from build123d import *

# Parameters (mm, degrees)
BOSS_EXTRUDE1_DEPTH      = 5
BOSS_EXTRUDE1_DEPTH_BACK = 5
SKETCH1_R                = 1.5
CUT_EXTRUDE1_DEPTH       = 5
SKETCH5_R                = 2.5
CUT_EXTRUDE3_DEPTH       = 30
SKETCH6_R                = 1.5
SKETCH6_R_2              = 1.843261337
CUT_EXTRUDE4_DEPTH       = 42


with BuildPart() as part:
    # Sketch1 → Boss-Extrude1 (new, two sides: drawn at the far end of the back side and taken through both)
    with BuildSketch(Plane(origin=(0, 0, 0), x_dir=(1, 0, 0), z_dir=(0, 1, 0)).offset(-BOSS_EXTRUDE1_DEPTH_BACK)):
        with BuildLine():
            Line((0, 17.525), (0, 40))
            Line((0, 40), (-36, 40))
            Line((-36, 40), (-36, -40))
            Line((-36, -40), (0, -40))
            Line((0, -40), (0, -17.525))
            ThreePointArc((0, -17.525), (-17.525, 0), (0, 17.525))
        make_face()
        with Locations(Location((-24.748737342, 24.748737342, 0), (0, 0, 270))):
            Circle(SKETCH1_R, mode=Mode.SUBTRACT)
        with Locations(Location((-24.748737342, -24.748737342, 0), (0, 0, 270))):
            Circle(SKETCH1_R, mode=Mode.SUBTRACT)
    extrude(amount=BOSS_EXTRUDE1_DEPTH + BOSS_EXTRUDE1_DEPTH_BACK)

    # Sketch2 → Cut-Extrude1 (cut)
    with BuildSketch(Plane(origin=(0, 5, 0), x_dir=(1, 0, 0), z_dir=(0, 1, 0))):
        Polygon((-23.161024101, 27.498737342), (-26.336450582, 27.498737342), (-27.924163822, 24.748737342), (-26.336450582, 21.998737342), (-23.161024101, 21.998737342), (-21.573310861, 24.748737342), align=None)
    cut_extrude1 = extrude(amount=-CUT_EXTRUDE1_DEPTH, mode=Mode.SUBTRACT)

    # Mirror1: Cut-Extrude1 across plane
    add(cut_extrude1.mirror(Plane.XY), mode=Mode.SUBTRACT)

    # Sketch5 → Cut-Extrude3 (cut)
    with BuildSketch(Plane.ZY.offset(36)):
        with Locations((-30, 0)):
            Circle(SKETCH5_R)
        Polygon((31.592573026, 2.747490689), (28.417151509, 2.753105152), (26.824578483, 0.005916682), (28.407426974, -2.746886251), (31.582848491, -2.752500714), (33.175421517, -0.005312244), align=None)
    extrude(amount=-CUT_EXTRUDE3_DEPTH, mode=Mode.SUBTRACT)

    # Sketch6 → Cut-Extrude4 (cut)
    with BuildSketch(Plane.ZY.offset(36)):
        with Locations((-30, 0)):
            Circle(SKETCH6_R)
        with Locations((30, 0)):
            Circle(SKETCH6_R_2)
    extrude(amount=-CUT_EXTRUDE4_DEPTH, mode=Mode.SUBTRACT)


solid = part.part
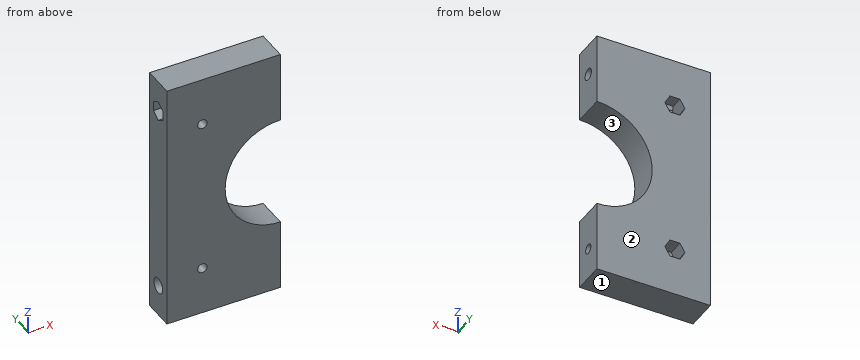
Source: CAD feature listing. Evaluate the final solid. Frame: model axes, mm. Face numbers are marked on the shaded views. Coordinates: 2 decimals unless noted, no trailing zeros. Order: outer loops, then holes, each group sorted by start corner. A loop starts at its lowest first (then second) coordinate and runs counter-clockwise, first axis right, second up.
Item 1: Pull-direction query (Z, two-part tool) for the marked faces 1, 2 and 3; classes: pulls with the +Z half, pulls with the -Z half, needs draft (parallel to the pull), parting line crosses it, or undercut.
Output values:
face 1: pulls with the -Z half
face 2: needs draft
face 3: undercut
Item 2: Cut plane B-B (z = -30). Return loops of the section in (x, y).
Output values:
outline: (-36, -5) - (0, -5) - (0, -1.5) - (-6, -1.5) - (-6, -2.5) - (-36, -2.5) - close; (-36, 2.5) - (-6, 2.5) - (-6, 1.5) - (0, 1.5) - (0, 5) - (-36, 5) - close
Item 3: Cut plane D-D (z = 0). Return loops of the section in (x, y) (3 decimals), plus the area to 3 significant figures.
Output values:
outline: (-36, -5) - (-17.525, -5) - (-17.525, 5) - (-36, 5) - close
area: 185 mm2
Item 4: Cut plane A-A (x = -7). Return loops of the section in (y, z).
Output values:
outline: (-5, -40) - (5, -40) - (5, -16.07) - (-5, -16.07) - close; (-5, 16.07) - (5, 16.07) - (5, 40) - (-5, 40) - close; hole (-2.75, 28.41) - (0.01, 26.82) - (2.75, 28.42) - (2.75, 31.59) - (-0.01, 33.18) - (-2.75, 31.58) - close; hole circle Ø5 at (0, -30)
Item 5: First-contact query: P1, Ø5, axis at x = -24.75, z = 24.75, coming from the -Y side; P2, Ø4, axis at y = 0, z = 30, coming from the -X side; P3, Ø6, axis at y = -2.5, z = 0.5, coming from the +X side; P4, Ø1.6, axis at x = -23.5, z = -26, coming from the +Y side. Flat tips, straight axial feed; report the tip coordinate or a pass-through.
Output values:
P1: stops at y = -5
P2: stops at x = -6
P3: stops at x = -17.17
P4: stops at y = 0
Item 6: Material intervals for line 1 (Y direction, x = -3.95, z = -30); line 2 (Z direction, x = -32, y = -1.5); line 3 (Y direction, x = -4.65, z = 30), sorted ascending.
Output values:
line 1: y = -5 to -1.5, 1.5 to 5
line 2: z = -40 to -32, -28 to 27.69, 32.31 to 40
line 3: y = -5 to -1.84, 1.84 to 5
Item 7: Cut plane C-C (x = -12). Return loops of the section in (y, z), plus the area to 3 significant figures.
Output values:
outline: (-5, -40) - (5, -40) - (5, -12.77) - (-5, -12.77) - close; (-5, 12.77) - (5, 12.77) - (5, 40) - (-5, 40) - close; hole (-2.75, 28.41) - (0.01, 26.82) - (2.75, 28.42) - (2.75, 31.59) - (-0.01, 33.18) - (-2.75, 31.58) - close; hole circle Ø5 at (0, -30)
area: 499 mm2
